Read the model definition and answer for the solid it produces. Units are mm, in the model's axes. A direction names the side the tool comes from. Round coordinates to 2 decimals unless told otherwise and drop trailing zeros. Order: outer loops, then holes, each group sorted by start corner. A loop starts at its lowest first (then second) coordinate and runs counter-clockwise, first axis right, second up. Notation, with made-up numbers: (77, 36.25) - (128, 36.25) arc R7 cw to (128, 41.25) - close; hole circle Ø2 at (36.25, 0). An arc over 180 degrees is marked (long way). Answer as a JSON object with one key per item and string values. Group by question number.
Q1. A cutting plane is placed at C-C on z = 1. Determine the outline of the cut face in (x, y).
Q2. A tool of negligible diameter and unlimited length cuts with its end or side. For faces 4 (the flat face through (3.133, -1.9, 2.5)), 5 (the flat face through (0, 0, 0)), from which of +Z, -Z, +X, -X, +Y, -Y can it reach the whole face along a straight path? Write none if from no direction.
Q3. A cutting plane is placed at D-D on x = -5.25. Determine the outline of the cut face in (y, z), and give its area (3 significant figures).
Q4. The mould has two halves that part along Y. Classify faces 1 (the flat face through (0, 8.2, 3)), 2 (the flat face through (-2.4, 4.624, 2.5)), 3 (the cylindrical face through (-2.17, -9.76, 1.48)): pulls with the +Y half, pulls with the -Y half, needs draft (parallel to the pull), parting line crosses it, or undercut.
Q5. Consider line 1 (Z direction, x = 5.5, y = -3.25); line 2 (X direction, y = 0.25, z = 1.8); line 3 (Y direction, x = -4.25, z = 2.55). Determine where each line is inside the solid, lowest interval first.
Q6. A cutting plane is placed at B-B on y = -5. Determine the outline of the cut face in (x, z) (3 decimals), and give its area (3 significant figures).
Q7. Given pin 1 Ø1.1 at (y, z) = (-1.5, 2.5) entering from -X; pin 2 Ø0.6 at (y, z) = (4, 2.5) entering from -X; pin 3 Ø1 at (y, z) = (-4, 2.5) entering from -X, each flat-ended and moving along its own axis, determine where each tip first touches the part or whether it passes through.
Q8. A cutting plane is placed at A-A on x = 7. Determine the outline of the cut face in (y, z), and give its area (3 significant figures).
```python
from build123d import *

# Parameters (mm, degrees)
SKETCH_1_R          = 10
EXTRUDE_1_DEPTH     = 3
SKETCH_2_R          = 8
CUT_EXTRUDE_1_DEPTH = 1
EXTRUDE_3_DEPTH     = 1


with BuildPart() as part:
    # 草图1 → 凸台-拉伸1 (new body)
    with BuildSketch(Plane.XY):
        Circle(SKETCH_1_R)
    extrude(amount=EXTRUDE_1_DEPTH)

    # 草图2 → 切除-拉伸1 (cut)
    with BuildSketch(Plane.XY.offset(3)):
        Circle(SKETCH_2_R)
    extrude(amount=-CUT_EXTRUDE_1_DEPTH, mode=Mode.SUBTRACT)

    # 草图4 → 凸台-拉伸3 (add)
    with BuildSketch(Plane.XY.offset(2)):
        with BuildLine():
            Line((0.056762987, 1.474211792), (-2.010233509, 1.474211792))
            Line((-2.010233509, 1.474211792), (-2.010233509, 1.80333177))
            add(Edge.make_bspline(
                [(-2.010233509, 1.80333177), (-2.010714949, 1.845366066), (-2.011636853, 1.925857174), (-2.013443384, 2.040830842), (-2.021934942, 2.144355468), (-2.031073109, 2.236120108), (-2.040588927, 2.31710552), (-2.056465146, 2.385691054), (-2.072751931, 2.443681195), (-2.098421022, 2.504945758), (-2.146218174, 2.567628601), (-2.227072107, 2.622444592), (-2.333658747, 2.649566324), (-2.411001767, 2.653311278), (-2.45316133, 2.655352647)],
                knots=[0, 0, 0, 0, 1.359919446, 2.604097865, 3.718258517, 4.718210111, 5.588312068, 6.352757529, 6.992875727, 7.535071206, 8.493600252, 9.496298216, 10.635235939, 12, 12, 12, 12], degree=3))
            add(Edge.make_bspline(
                [(-2.45316133, 2.655352647), (-2.48769324, 2.653727226), (-2.553890817, 2.650611298), (-2.646642148, 2.622991559), (-2.725077805, 2.574799662), (-2.789460033, 2.508992999), (-2.837678653, 2.423435949), (-2.872664288, 2.321405275), (-2.891615661, 2.200286181), (-2.894528446, 2.114059415), (-2.89608915, 2.067858107)],
                knots=[0, 0, 0, 0, 0.988105774, 1.894196063, 2.738146432, 3.600308196, 4.502221556, 5.528881054, 6.675945596, 8, 8, 8, 8], degree=3))
            add(Edge.make_bspline(
                [(-2.89608915, 2.067858107), (-2.894449613, 1.992202619), (-2.891412238, 1.85204466), (-2.851820774, 1.660792354), (-2.795166347, 1.499557252), (-2.727751468, 1.419469509), (-2.696156454, 1.381935163)],
                knots=[0, 0, 0, 0, 1.238590262, 2.294589406, 3.200733242, 4, 4, 4, 4], degree=3))
            add(Edge.make_bspline(
                [(-2.696156454, 1.381935163), (-2.676461776, 1.363134012), (-2.630861227, 1.319602312), (-2.545176258, 1.255053383), (-2.437113188, 1.178219265), (-2.306005051, 1.088728044), (-2.150665321, 0.987994219), (-1.972415244, 0.873613916), (-1.769467583, 0.749717147), (-1.625830171, 0.664089009), (-1.550388307, 0.619115027)],
                knots=[0, 0, 0, 0, 0.473750368, 1.096909409, 1.864751644, 2.783261057, 3.860202471, 5.088360878, 6.470736284, 8, 8, 8, 8], degree=3))
            add(Edge.make_bspline(
                [(-1.550388307, 0.619115027), (-1.485198527, 0.580292401), (-1.360104373, 0.505794778), (-1.181709189, 0.396565598), (-1.019465077, 0.294906955), (-0.873253022, 0.199660286), (-0.743042002, 0.110905609), (-0.629062244, 0.029561017), (-0.531324757, -0.044462306), (-0.421492641, -0.134926314), (-0.298119069, -0.256239512), (-0.16776821, -0.425307224), (-0.049470339, -0.620618928), (0.056905891, -0.841480009), (0.147481943, -1.089394), (0.208560212, -1.367548532), (0.2478522, -1.673343211), (0.251643957, -1.887086396), (0.253619796, -1.998465357)],
                knots=[0, 0, 0, 0, 1.071987144, 2.057060554, 2.955337459, 3.77699406, 4.522318602, 5.181589955, 5.755251306, 6.254177214, 7.191438167, 8.192596657, 9.262134101, 10.412151394, 11.651634359, 12.981704702, 14.427203216, 16, 16, 16, 16], degree=3))
            add(Edge.make_bspline(
                [(0.253619796, -1.998465357), (0.252520604, -2.088771103), (0.250373462, -2.265172779), (0.222764294, -2.521443005), (0.18288396, -2.763633873), (0.12157342, -2.989934303), (0.048224142, -3.203329396), (-0.04764749, -3.399426406), (-0.155935901, -3.582886354), (-0.284918565, -3.748769407), (-0.428419819, -3.901762054), (-0.591566185, -4.036202813), (-0.768685194, -4.159846558), (-0.965671944, -4.262796907), (-1.17743885, -4.354992249), (-1.406900356, -4.429013379), (-1.652957644, -4.490181019), (-1.823878665, -4.516421874), (-1.911805105, -4.529920886)],
                knots=[0, 0, 0, 0, 1.166783885, 2.279175364, 3.328322562, 4.336159768, 5.306592857, 6.240240115, 7.152837026, 8.055466775, 8.95076907, 9.858637968, 10.783210379, 11.737857823, 12.726337121, 13.765749244, 14.850640409, 16, 16, 16, 16], degree=3))
            Line((-1.911805105, -4.529920886), (-1.911805105, -5.317348123))
            Line((-1.911805105, -5.317348123), (-2.89608915, -5.317348123))
            Line((-2.89608915, -5.317348123), (-2.89608915, -4.529920886))
            add(Edge.make_bspline(
                [(-2.89608915, -4.529920886), (-2.964444513, -4.521229842), (-3.099464254, -4.504062754), (-3.297451441, -4.460222183), (-3.489345523, -4.402463406), (-3.673272398, -4.325457939), (-3.853248014, -4.239077881), (-4.024367639, -4.13315523), (-4.188527464, -4.012378649), (-4.349076156, -3.880100488), (-4.495366504, -3.723540065), (-4.622435632, -3.53984494), (-4.72817515, -3.328806901), (-4.813652178, -3.091543394), (-4.880733234, -2.828813828), (-4.929378662, -2.540298927), (-4.958678767, -2.225151111), (-4.961577762, -2.006221367), (-4.963085646, -1.892347233)],
                knots=[0, 0, 0, 0, 0.880722716, 1.739658008, 2.589843307, 3.439548281, 4.286822195, 5.140160776, 6.008178737, 6.892018721, 7.796500557, 8.738476021, 9.73819386, 10.806244783, 11.957388676, 13.201071447, 14.544165091, 16, 16, 16, 16], degree=3))
            Line((-4.963085646, -1.892347233), (-4.963085646, -1.478640345))
            Line((-4.963085646, -1.478640345), (-2.89608915, -1.478640345))
            Line((-2.89608915, -1.478640345), (-2.89608915, -1.992313581))
            add(Edge.make_bspline(
                [(-2.89608915, -1.992313581), (-2.895704026, -2.059471516), (-2.894971956, -2.187129782), (-2.891957149, -2.369133466), (-2.88733937, -2.53113795), (-2.881948967, -2.673237924), (-2.87257906, -2.794763684), (-2.861999559, -2.896309089), (-2.850782323, -2.978298671), (-2.831771987, -3.057698517), (-2.796329914, -3.13720338), (-2.724733914, -3.204634246), (-2.630260737, -3.245729545), (-2.560258212, -3.248728448), (-2.522368802, -3.250351627)],
                knots=[0, 0, 0, 0, 1.657418857, 3.150531957, 4.492147425, 5.657201955, 6.659563487, 7.499257938, 8.177392906, 8.69903519, 9.513866485, 10.283438363, 11.070897696, 12, 12, 12, 12], degree=3))
            add(Edge.make_bspline(
                [(-2.522368802, -3.250351627), (-2.489378542, -3.248660536), (-2.426843431, -3.245454967), (-2.339218716, -3.219229643), (-2.266135459, -3.173231759), (-2.207216552, -3.10880944), (-2.162940532, -3.026750233), (-2.13130144, -2.928258661), (-2.111154143, -2.813357435), (-2.109526388, -2.731132497), (-2.108661914, -2.687464189)],
                knots=[0, 0, 0, 0, 0.994883323, 1.88586392, 2.727487039, 3.570816153, 4.492326284, 5.520132617, 6.682983341, 8, 8, 8, 8], degree=3))
            add(Edge.make_bspline(
                [(-2.108661914, -2.687464189), (-2.108935574, -2.631069741), (-2.10946309, -2.52236181), (-2.114071505, -2.36544721), (-2.121638763, -2.220834196), (-2.132025717, -2.088463373), (-2.146270394, -1.969077806), (-2.160677831, -1.861524675), (-2.180587972, -1.767054101), (-2.204007286, -1.681855361), (-2.2351748, -1.60114895), (-2.282906179, -1.522964225), (-2.34325911, -1.442242229), (-2.419461819, -1.361342915), (-2.508937636, -1.278209236), (-2.613142538, -1.193590203), (-2.730821056, -1.105545843), (-2.817259718, -1.050516127), (-2.862254386, -1.02187103)],
                knots=[0, 0, 0, 0, 1.380366004, 2.660842346, 3.842046573, 4.924766116, 5.910024558, 6.784900421, 7.579810868, 8.270991265, 8.946735927, 9.689207242, 10.50484436, 11.410582145, 12.404987482, 13.492712756, 14.694859961, 16, 16, 16, 16], degree=3))
            add(Edge.make_bspline(
                [(-2.862254386, -1.02187103), (-2.937220205, -0.973865027), (-3.081396493, -0.881538587), (-3.286891769, -0.745807), (-3.474986034, -0.622159308), (-3.642992295, -0.505822423), (-3.79311186, -0.400793853), (-3.924056333, -0.305001794), (-4.036890963, -0.220601901), (-4.163849408, -0.119869901), (-4.304983023, 0.014315539), (-4.456319758, 0.199792286), (-4.595950479, 0.413669622), (-4.724454675, 0.652864388), (-4.833140109, 0.915678198), (-4.906897048, 1.199845959), (-4.95494887, 1.499747864), (-4.960333437, 1.705735293), (-4.963085646, 1.811021489)],
                knots=[0, 0, 0, 0, 1.144251925, 2.200656203, 3.165654651, 4.037535326, 4.827334008, 5.520628553, 6.122925727, 6.638522573, 7.603341009, 8.619197825, 9.708488222, 10.881837927, 12.105530735, 13.353920843, 14.647511608, 16, 16, 16, 16], degree=3))
            add(Edge.make_bspline(
                [(-4.963085646, 1.811021489), (-4.961832651, 1.886969132), (-4.959387355, 2.035185564), (-4.933923027, 2.250632635), (-4.894562266, 2.45413148), (-4.83767485, 2.644637628), (-4.765374936, 2.823312376), (-4.675972901, 2.98828905), (-4.570048913, 3.140778425), (-4.448675351, 3.280849467), (-4.310302398, 3.408108551), (-4.155692946, 3.521790754), (-3.985325259, 3.623865012), (-3.798953475, 3.712921544), (-3.595929506, 3.788193762), (-3.377284846, 3.850499543), (-3.14270702, 3.902314827), (-2.979857079, 3.92384636), (-2.89608915, 3.934921906)],
                knots=[0, 0, 0, 0, 1.100217239, 2.147140655, 3.139410829, 4.100827409, 5.023841391, 5.928095608, 6.81431441, 7.709642577, 8.608754423, 9.533023434, 10.486107416, 11.483039549, 12.522183369, 13.62029137, 14.775908296, 16, 16, 16, 16], degree=3))
            Line((-2.89608915, 3.934921906), (-2.89608915, 4.623920738))
            Line((-2.89608915, 4.623920738), (-1.911805105, 4.623920738))
            Line((-1.911805105, 4.623920738), (-1.911805105, 3.934921906))
            add(Edge.make_bspline(
                [(-1.911805105, 3.934921906), (-1.83113698, 3.923684787), (-1.674057582, 3.90180353), (-1.447521608, 3.852095654), (-1.236442357, 3.791447846), (-1.041243092, 3.71680636), (-0.860526928, 3.631897354), (-0.697329997, 3.531284043), (-0.5494265, 3.419578532), (-0.416662802, 3.296239572), (-0.298135254, 3.160524603), (-0.199220323, 3.009701153), (-0.111370998, 2.849607494), (-0.042910487, 2.675016965), (0.012954, 2.489539125), (0.050711945, 2.290569889), (0.074127815, 2.080216319), (0.07688497, 1.935659253), (0.0782942, 1.861773635)],
                knots=[0, 0, 0, 0, 1.217065147, 2.369905846, 3.463567771, 4.496793418, 5.490769135, 6.443602658, 7.357042595, 8.257109579, 9.148127797, 10.042894642, 10.948036131, 11.87297517, 12.840365016, 13.839761067, 14.895864502, 16, 16, 16, 16], degree=3))
            add(Edge.make_bspline(
                [(0.0782942, 1.861773635), (0.077810751, 1.837679646), (0.076740765, 1.784353921), (0.074244937, 1.695560092), (0.065389733, 1.590583694), (0.059765481, 1.514714431), (0.056762987, 1.474211792)],
                knots=[0, 0, 0, 0, 0.744858199, 1.648548241, 2.744682654, 4, 4, 4, 4], degree=3))
        make_face()
        with BuildLine():
            Line((5.023175077, 3.083267731), (5.023175077, -3.688606503))
            Line((5.023175077, -3.688606503), (3.133349709, -3.688606503))
            Line((3.133349709, -3.688606503), (3.133349709, -0.049216244))
            add(Edge.make_bspline(
                [(3.133349709, -0.049216244), (3.133593958, 0.010662586), (3.134055716, 0.123864492), (3.130999708, 0.284214806), (3.128343293, 0.425283899), (3.127055881, 0.546751118), (3.121323717, 0.64841284), (3.116976452, 0.730915963), (3.111457202, 0.794221383), (3.102291906, 0.852121983), (3.083359365, 0.90808358), (3.047418069, 0.964547564), (2.998087245, 1.01190667), (2.94587648, 1.044463224), (2.893097842, 1.065050405), (2.840089727, 1.077930703), (2.775346455, 1.090596163), (2.697463576, 1.098009477), (2.607659433, 1.105428465), (2.505139966, 1.112148942), (2.390217008, 1.113575298), (2.30942017, 1.114313637), (2.267179749, 1.11469964)],
                knots=[0, 0, 0, 0, 1.950419782, 3.687300443, 5.223822311, 6.546637084, 7.643380878, 8.540030222, 9.237904201, 9.712291202, 10.447402628, 11.144124893, 11.871548827, 12.657464658, 13.131287025, 13.711290926, 14.431812681, 15.278611421, 16.257109778, 17.367920147, 18.623954072, 20, 20, 20, 20], degree=3))
            Line((2.267179749, 1.11469964), (2.030951578, 1.11469964))
            Line((2.030951578, 1.11469964), (2.030951578, 2.023932027))
            add(Edge.make_bspline(
                [(2.030951578, 2.023932027), (2.130150393, 2.047183275), (2.324590782, 2.092758233), (2.604092231, 2.182654867), (2.864873324, 2.289383591), (3.106344693, 2.414498141), (3.329490435, 2.555636371), (3.533824466, 2.714185), (3.720026359, 2.888796928), (3.828520908, 3.018549566), (3.882635939, 3.083267731)],
                knots=[0, 0, 0, 0, 1.122506737, 2.20023443, 3.231784783, 4.224338166, 5.193566431, 6.137412817, 7.070976693, 8, 8, 8, 8], degree=3))
            Line((3.882635939, 3.083267731), (5.023175077, 3.083267731))
        make_face()
    extrude(amount=EXTRUDE_3_DEPTH)


solid = part.part
```
Result set:
{
 "1": {"outline": "circle Ø20 at (0, 0)"},
 "2": {"face 4": "+Z", "face 5": "-Z, +X, -X, +Y, -Y"},
 "3": {"outline": "(-8.51, 0) - (8.51, 0) - (8.51, 3) - (6.04, 3) - (6.04, 2) - (-6.04, 2) - (-6.04, 3) - (-8.51, 3) - close", "area": "39.0 mm²"},
 "4": {"face 1": "needs draft", "face 2": "undercut", "face 3": "parting line crosses it"},
 "5": {"line 1": "z = 0 to 2", "line 2": "x = -10 to 10", "line 3": "y = -9.05 to -6.78, -3.96 to -1.48, -0.04 to 3.45, 6.78 to 9.05"},
 "6": {"outline": "(-8.66, 0) - (8.66, 0) - (8.66, 3) - (6.245, 3) - (6.245, 2) - (-1.912, 2) - (-1.912, 3) - (-2.896, 3) - (-2.896, 2) - (-6.245, 2) - (-6.245, 3) - (-8.66, 3) - close", "area": "40.5 mm²"},
 "7": {"pin 1": "stops at x = -9.95", "pin 2": "stops at x = -9.29", "pin 3": "stops at x = -9.37"},
 "8": {"outline": "(-7.14, 0) - (7.14, 0) - (7.14, 3) - (3.87, 3) - (3.87, 2) - (-3.87, 2) - (-3.87, 3) - (-7.14, 3) - close", "area": "35.1 mm²"}
}
